Model file for the job. Use its own axes, mm. A direction names the side the tool comes from. Round coordinates to 2 decimals unless told otherwise and drop trailing zeros. Loops run counter-clockwise (first coordinate to the right, second up) from the corner with the lowest first, then second, coordinate; pieces in that order, holes last. Notation, with made-up numbers: (45, 28) -> (80, 28) arc R20 ccw to (80, 58) -> close; hole circle Ø3 at (-19, 31.5). An arc over 180 degrees is marked (long way). Use a Markdown table: item, result.
from build123d import *

# Parameters (mm, degrees)
SKETCH_W        = 25
SKETCH_H        = 50
PAD_DEPTH       = 78
SKETCH001_W     = 10
SKETCH001_H     = 30
POCKET_DEPTH    = 50
SKETCH002_W     = 20
SKETCH002_H     = 48
PAD001_DEPTH    = 49
FILLET_R        = 24
POCKET001_DEPTH = 20
SKETCH004_W     = 50
SKETCH004_H     = 15
PAD002_DEPTH    = 60
FILLET001_R     = 25
POCKET002_DEPTH = 15
SKETCH006_R     = 12
POCKET003_DEPTH = 20
POCKET004_DEPTH = 15
POCKET005_DEPTH = 15
POCKET006_DEPTH = 25
PAD003_DEPTH    = 10
PAD004_DEPTH    = 10


with BuildPart() as part:
    # Sketch → Pad (new body)
    with BuildSketch(Plane.XY):
        with Locations((12.5, 25)):
            Rectangle(SKETCH_W, SKETCH_H)
    extrude(amount=PAD_DEPTH)

    # Sketch001 (on Face3 of Pad) → Pocket (cut)
    with BuildSketch(Plane(origin=(0, 50, 0), x_dir=(-1, 0, 0), z_dir=(0, 1, 0))):
        with Locations((-5, 63)):
            Rectangle(SKETCH001_W, SKETCH001_H)
    extrude(amount=-POCKET_DEPTH, mode=Mode.SUBTRACT)

    # Sketch002 (on Face7 of Pocket) → Pad001 (join)
    with BuildSketch(Plane(origin=(0, 0, 0), x_dir=(0, -1, 0), z_dir=(-1, 0, 0))):
        with Locations((-10, 24)):
            Rectangle(SKETCH002_W, SKETCH002_H)
    extrude(amount=PAD001_DEPTH)

    # Fillet
    fillet_edges = [part.edges().sort_by_distance(p)[0] for p in [
        (-49, 10, 0),
    ]]
    fillet(fillet_edges, radius=FILLET_R)

    # Sketch003 (on Face8 of Fillet) → Pocket001 (cut)
    with BuildSketch(Plane(origin=(0, 20, 0), x_dir=(-1, 0, 0), z_dir=(0, 1, 0))):
        with BuildLine():
            ThreePointArc((49, 24), (41.970563, 40.970563), (25, 48))
            Line((25, 48), (49, 48))
            Line((49, 48), (49, 24))
        make_face()
    extrude(amount=-POCKET001_DEPTH, mode=Mode.SUBTRACT)

    # Sketch004 (on Face10 of Pocket001) → Pad002 (join)
    with BuildSketch(Plane.YZ.offset(25)):
        with Locations((25, 70.5)):
            Rectangle(SKETCH004_W, SKETCH004_H)
    extrude(amount=PAD002_DEPTH)

    # Fillet001
    fillet001_edges = [part.edges().sort_by_distance(p)[0] for p in [
        (85, 0, 70.5),
    ]]
    fillet(fillet001_edges, radius=FILLET001_R)

    # Sketch005 (on Face2 of Fillet001) → Pocket002 (cut)
    with BuildSketch(Plane.XY.offset(78)):
        with BuildLine():
            ThreePointArc((85, 25), (77.67767, 42.67767), (60, 50))
            Line((60, 50), (85, 50))
            Line((85, 50), (85, 25))
        make_face()
    extrude(amount=-POCKET002_DEPTH, mode=Mode.SUBTRACT)

    # Sketch006 (on Face20 of Pocket002) → Pocket003 (cut)
    with BuildSketch(Plane(origin=(0, 20, 0), x_dir=(-1, 0, 0), z_dir=(0, 1, 0))):
        with Locations((25, 24)):
            Circle(SKETCH006_R)
    extrude(amount=-POCKET003_DEPTH, mode=Mode.SUBTRACT)

    # Sketch007 (on Face2 of Pocket003) → Pocket004 (cut)
    with BuildSketch(Plane.XY.offset(78)):
        with BuildLine():
            ThreePointArc((60, 12), (73, 25), (60, 38))
            Line((60, 38), (36, 38))
            Line((36, 38), (36, 12))
            Line((36, 12), (60, 12))
        make_face()
    extrude(amount=-POCKET004_DEPTH, mode=Mode.SUBTRACT)

    # Sketch008 (on Face15 of Pocket004) → Pocket005 (cut)
    with BuildSketch(Plane(origin=(10, 0, 0), x_dir=(0, -1, 0), z_dir=(-1, 0, 0))):
        with BuildLine():
            ThreePointArc((-33, 61), (-38, 56), (-33, 51))
            Line((-33, 51), (-17, 51))
            ThreePointArc((-17, 51), (-12, 56), (-17, 61))
            Line((-33, 61), (-17, 61))
        make_face()
    extrude(amount=-POCKET005_DEPTH, mode=Mode.SUBTRACT)

    # Sketch009 (on Face19 of Pocket005) → Pocket006 (cut)
    with BuildSketch(Plane(origin=(0, 0, 0), x_dir=(0, -1, 0), z_dir=(-1, 0, 0))):
        with BuildLine():
            ThreePointArc((-35, 14), (-30, 9), (-25, 14))
            Line((-25, 14), (-25, 34))
            ThreePointArc((-25, 34), (-30, 39), (-35, 34))
            Line((-35, 14), (-35, 34))
        make_face()
    extrude(amount=-POCKET006_DEPTH, mode=Mode.SUBTRACT)

    # Sketch010 (on DatumPlane) → Pad003 (join)
    with BuildSketch(Plane.XZ):
        with BuildLine():
            Line((10, 48), (10, 78))
            Line((10, 78), (-38.818227, 43.622859))
            ThreePointArc((-25, 48), (-32.247461, 46.879561), (-38.818227, 43.622859))
            Line((10, 48), (-25, 48))
        make_face()
    extrude(amount=-PAD003_DEPTH)

    # Sketch011 (on DatumPlane) → Pad004 (join)
    with BuildSketch(Plane(origin=(0, 50, 0), x_dir=(-1, 0, 0), z_dir=(0, 1, 0))):
        Polygon((-60, 63), (-25, 63), (-25, 0), align=None)
    extrude(amount=-PAD004_DEPTH)


solid = part.part
Q1. Tool access for faces 1 (the face through (12, 35, 24)), 2 (the face through (1, 26, 48)), 3 (the face through (36, 25, 71)): list every direction of +Z, -Z, +X, -X, +Y, -Y with a clear straight run to the whole face (end or side of a thin tool).
Results list:
| item | result |
|---|---|
| face 1 | +X, -X |
| face 2 | +Z, -X, +Y |
| face 3 | +Z, -Z |
Q2. Band-saw the part on C-C, the plane y = 30. Give the cut face in (x, z).
Results list:
| item | result |
|---|---|
| outline | (0, 0) -> (25, 0) -> (25, 9) -> (0, 9) -> close; (0, 39) -> (25, 39) -> (25, 51) -> (10, 51) -> (10, 48) -> (0, 48) -> close; (10, 61) -> (25, 61) -> (25, 63) -> (36, 63) -> (36, 78) -> (10, 78) -> close; (72, 63) -> (84.49, 63) -> (84.49, 78) -> (72, 78) -> close |
Q3. Pull direction Y, two halves, no side cores. Call faces 4 (the face through (17, 25, 61)), 5 (the face through (-14.07, 4.93, 61.05)), 6 (the face through (73, 25, 71)), 7 (the face through (38, 40, 39)): released by +Y, released by -Y, zero draft, split by the parting line, or undercut.
Results list:
| item | result |
|---|---|
| face 4 | undercut |
| face 5 | zero draft |
| face 6 | undercut |
| face 7 | released by -Y |
Q4. Band-saw the part on B-B, the plane z = 26.5. Give the cut face in (x, y), plus the area to 3 significant figures.
Results list:
| item | result |
|---|---|
| outline | (-48.87, 0) -> (-36.74, 0) -> (-36.74, 20) -> (-48.87, 20) -> close; (-13.26, 0) -> (25, 0) -> (25, 25) -> (0, 25) -> (0, 20) -> (-13.26, 20) -> close; (0, 35) -> (25, 35) -> (25, 40) -> (39.72, 40) -> (39.72, 50) -> (0, 50) -> close |
| area | 1,660 mm² |
Q5. Band-saw the part on D-D, the plane x = 22.5. Give the cut face in (y, z), plus the area to 3 significant figures.
Results list:
| item | result |
|---|---|
| outline | (0, 0) -> (50, 0) -> (50, 78) -> (0, 78) -> close; hole (17, 51) -> (33, 51) arc R5 ccw to (33, 61) -> (17, 61) arc R5 ccw to start; hole (25, 14) arc R5 ccw to (35, 14) -> (35, 34) arc R5 ccw to (25, 34) -> close |
| area | 3,380 mm² |
Q6. Band-saw the part on A-A, the plane x = 40. Give the cut face in (y, z).
Results list:
| item | result |
|---|---|
| outline | (0, 63) -> (12, 63) -> (12, 78) -> (0, 78) -> close; (38, 63) -> (40, 63) -> (40, 27) -> (50, 27) -> (50, 78) -> (38, 78) -> close |
Q7. Flat gauge pins, fed straight in: pin 1 (10 mm diameter, centred on x = 36.5, y = 31, fed in from -Z); pin 2 (10 mm diameter, centred on y = 27, z = 14.5, fed in from -X); pin 3 (10 mm diameter, centred on x = 45.5, y = 42, fed in from -Z). Where does each tip first touch, or does it go through?
Results list:
| item | result |
|---|---|
| pin 1 | stops at z = 63 |
| pin 2 | stops at x = 0 |
| pin 3 | stops at z = 27.9 |
Q8. Drill centre lines: L1, parallel to Z at x = -25, y = 12; L2, parallel to Z at x = 23, y = 26; L3, parallel to X at y = 38, z = 25. Where is each one in solid material? Low to high. Write a range as from..to.
Results list:
| item | result |
|---|---|
| L1 | z = 0..12, 36..48 |
| L2 | z = 0..11, 37..51, 61..78 |
| L3 | x = 0..25 |
